from build123d import *

# Parameters (mm, degrees)
SKETCH1_W                 = 63.5
SKETCH1_H                 = 63.5
BOSS_EXTRUDE1_DEPTH       = 3.175
BOSS_EXTRUDE2_DEPTH       = 4.7625
F_2_CLEARANCE_HOLE2_D     = 2.4384
F_2_CLEARANCE_HOLE2_DEPTH = 3.155006513
FILLET1_R                 = 19.05
SKETCH7_W                 = 15.875
SKETCH7_H                 = 3.175
BOSS_EXTRUDE3_DEPTH       = 4.7625
F_2_CLEARANCE_HOLE3_D     = 2.4384
F_2_CLEARANCE_HOLE3_DEPTH = 3.175
BOSS_EXTRUDE4_START       = -3.175
SKETCH10_R                = 3.175
BOSS_EXTRUDE4_DEPTH       = 3.175
F_6_CLEARANCE_HOLE1_D     = 3.7973
SKETCH13_R                = 3.175
CUT_EXTRUDE1_DEPTH        = 3.175


with BuildPart() as part:
    # Sketch1 → Boss-Extrude1 (new body)
    with BuildSketch(Plane.XY):
        Rectangle(SKETCH1_W, SKETCH1_H)
    extrude(amount=BOSS_EXTRUDE1_DEPTH)

    # Sketch2 → Boss-Extrude2 (add)
    with BuildSketch(Plane(origin=(0, 0, 0), x_dir=(-1, 0, 0), z_dir=(0, 0, -1))):
        Polygon((15.875, -31.75), (25.4, -31.75), (31.75, -31.75), (31.75, -28.594993487), (25.755751185, -28.594993487), (15.875, -28.594993487), align=None)
    extrude(amount=BOSS_EXTRUDE2_DEPTH)

    # #2 Clearance Hole2
    with Locations(Plane(origin=(0, -28.594993487, 0), x_dir=(1, 0, 0), z_dir=(0, 1, 0))):
        with Locations((-28.575, 2.447629477), (-19.05, 2.447629477)):
            Hole(F_2_CLEARANCE_HOLE2_D / 2, depth=F_2_CLEARANCE_HOLE2_DEPTH)

    # Fillet1
    fillet1_edges = [part.edges().sort_by_distance(p)[0] for p in [
        (31.75, -31.75, 1.5875),
        (31.75, 31.75, 1.5875),
    ]]
    fillet(fillet1_edges, radius=FILLET1_R)

    # Sketch7 → Boss-Extrude3 (add)
    with BuildSketch(Plane(origin=(0, 0, 0), x_dir=(-1, 0, 0), z_dir=(0, 0, -1))):
        with Locations((23.8125, 30.1625)):
            Rectangle(SKETCH7_W, SKETCH7_H)
    extrude(amount=BOSS_EXTRUDE3_DEPTH)

    # #2 Clearance Hole3
    with Locations(Plane(origin=(0, 31.75, 0), x_dir=(1, 0, 0), z_dir=(0, 1, 0))):
        with Locations((-28.575, 2.447629477), (-19.05, 2.447629477)):
            Hole(F_2_CLEARANCE_HOLE3_D / 2, depth=F_2_CLEARANCE_HOLE3_DEPTH)

    # Sketch10 → Boss-Extrude4 (add)
    with BuildSketch(Plane.XY.offset(3.175).offset(BOSS_EXTRUDE4_START)):
        with Locations((25.4, 19.05)):
            Circle(SKETCH10_R)
        with Locations((-22.225, 19.05)):
            Circle(SKETCH10_R)
        with Locations((-22.225, -14.2875)):
            Circle(SKETCH10_R)
        with Locations((-8.73125, -24.209375)):
            Circle(SKETCH10_R)
        with Locations((11.90625, -24.209375)):
            Circle(SKETCH10_R)
    extrude(amount=-BOSS_EXTRUDE4_DEPTH)

    # #6 Clearance Hole1 (through all)
    with Locations(Plane(origin=(0, 0, -3.175), x_dir=(-1, 0, 0), z_dir=(0, 0, -1))):
        with Locations((-25.4, 19.05), (22.225, 19.05), (22.225, -14.2875), (8.73125, -24.209375), (-11.90625, -24.209375)):
            Hole(F_6_CLEARANCE_HOLE1_D / 2)

    # Sketch13 → Cut-Extrude1 (cut)
    with BuildSketch(Plane.XY.offset(3.175)):
        with Locations((1.5875, -23.415625)):
            Circle(SKETCH13_R)
        with BuildLine():
            Line((-1.5875, 23.01875), (4.7625, 23.01875))
            ThreePointArc((4.7625, 23.01875), (15.875, 11.90625), (4.7625, 0.79375))
            Line((4.7625, 0.79375), (-1.5875, 0.79375))
            ThreePointArc((-1.5875, 0.79375), (-12.7, 11.90625), (-1.5875, 23.01875))
        make_face()
    extrude(amount=-CUT_EXTRUDE1_DEPTH, mode=Mode.SUBTRACT)


solid = part.part
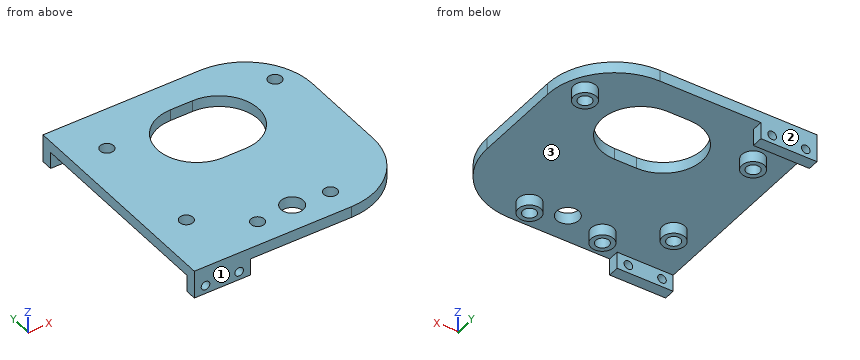
Geometry: final body of the model. Coordinates: model frame, mm. Face numbers are marked on the shaded views. Give positions to 0.01 mm unless a question says otherwise; leave off trailing zeros. Write each loop counter-clockwise with the first axis right and the second up, starting at its lowest first coordinate (ties: lowest second). Pieces come first, ordered by that corner, then holes. Notation, with made-up numbers: M 84,-39.75 L 143,-39.75 A16 cw 143,-22.75 Z; hole C 2,-39.5 d1. An arc over 180 degrees is marked long. Answer in a Markdown table with one row per item. Add a question column.
(1) Section C-C on z = 0.75. State how many separate pieces and enclosed holes the cut face has, and give its area (3 significant figures).
(2) First-contact query: pin 1 (2 mm diameter, centred on x = -19.05, z = -2.45, fed in from -Y); pin 2 (5 mm diameter, centred on x = -22, y = -14.5, fed in from -Z) (3 decimals); pin 3 (1 mm diameter, centred on y = 31, z = -2, fed in from +X) (3 decimals). Flat tips, straight axial feed; report the tip coordinate or a pass-through.
(3) Mould query, pull axis Y, two halves, no side actions, for the marked faces 1, 2 and 3. Classes: +Y half, -Y half, draft (parallel to the pull), parting line (faces both ways), or undercut.
(4) Section A-A on y = 19.05. Return loops of the section in (x, z) (3 decimals), and give its area (3 significant figures).
(5) Section B-B on x = 25.4. Return loops of the section in (y, z) (3 decimals), and give its area (3 significant figures).
(6) Section D-D on x = -14. Return loops of the section in (y, z) (3 decimals), and give its area (3 significant figures).
(7) Ray query, line 1 (Y direction, x = -23.5, z = -0.5) (3 decimals); line 2 (Y direction, x = 13, z = 2.75); line 3 (X direction, y = 20.5, z = 1.5). Return the intervals inside material, ascending.
Result set:
| question | item | result |
|---|---|---|
| 1 | separate pieces | 1 |
| 1 | enclosed holes | 7 |
| 1 | area | 3,260 mm^2 |
| 2 | pin 1 | stops at y = -16.6 |
| 2 | pin 2 | stops at z = -3.175 |
| 2 | pin 3 | stops at x = -15.875 |
| 3 | face 1 | -Y half |
| 3 | face 2 | +Y half |
| 3 | face 3 | undercut |
| 4 | outline | M -31.75,0 L -25.4,0 L -25.4,-3.175 L -24.124,-3.175 L -24.124,3.175 L -31.75,3.175 Z; M -20.326,-3.175 L -19.05,-3.175 L -19.05,0 L -10.1,0 L -10.1,3.175 L -20.326,3.175 Z; M 13.275,0 L 22.225,0 L 22.225,-3.175 L 23.501,-3.175 L 23.501,3.175 L 13.275,3.175 Z; M 27.299,-3.175 L 28.575,-3.175 L 28.575,0 L 30.661,0 L 30.661,3.175 L 27.299,3.175 Z |
| 4 | area | 116 mm^2 |
| 5 | outline | M -26.899,0 L 15.875,0 L 15.875,-3.175 L 17.151,-3.175 L 17.151,3.175 L -26.899,3.175 Z; M 20.949,-3.175 L 22.225,-3.175 L 22.225,0 L 26.899,0 L 26.899,3.175 L 20.949,3.175 Z |
| 5 | area | 167 mm^2 |
| 6 | outline | M -31.75,0 L 31.75,0 L 31.75,3.175 L -31.75,3.175 Z |
| 6 | area | 202 mm^2 |
| 7 | line 1 | y = -31.75 to -28.595, -17.195 to -15.694, -12.881 to -11.38, 16.142 to 17.643, 20.457 to 21.958, 28.575 to 31.75 |
| 7 | line 2 | y = -31.75 to -25.76, -22.66 to 4.45, 19.36 to 31.75 |
| 7 | line 3 | x = -31.75 to -23.45, -21 to -8.63, 11.81 to 24.17, 26.63 to 30.08 |
